Input: part model. Units: mm. Frame: model coordinates. A direction names the side the tool comes from. Round coordinates to 2 decimals unless told otherwise and drop trailing zeros. Loops run counter-clockwise (first coordinate to the right, second up) from the corner with the lowest first, then second, coordinate; pieces in that order, holes last. Notation, with made-up numbers: (0, 41) -> (34, 41) arc R7 cw to (34, 46) -> close; hole circle Ø1 at (36, 67.25). An arc over 180 degrees is marked (long way). Answer in a Markdown table with one row per item. Add a question column.
Q1. Ray query, L1, parallel to X at y = 61, z = 1; L2, parallel to Y at x = 25, z = 1.5; L3, parallel to Y at x = -42, z = 1.45. Return the intervals inside material, ascending. Write a range as from..to.
Q2. Section C-C, the plane y = 11.5. Output: boundary loops of the cut face in (x, z).
Q3. Section B-B, the plane y = 61.25. Output: boundary loops of the cut face in (x, z), and give its area (3 significant figures).
Q4. Mould query, pull axis Z, two halves, no side actions, for faces 1 (the face through (-11.15, -6.68, 25.87)), 2 (the face through (-30, 15, 25)), 3 (the face through (-26, 50, 5)). Classes: pulls with the +Z half, pulls with the -Z half, needs draft (parallel to the pull), parting line crosses it, or undercut.
Q5. Section D-D, the plane x = 15. Output: boundary loops of the cut face in (y, z).
Q6. Section A-A, the plane x = -10. Output: boundary loops of the cut face in (y, z).
Q7. Reachability of faces 4 (the face through (-67, 20, 2)), 5 (the face through (-17, 70, 7)), 6 (the face through (-75, 75, 2)) from +Z, -Z, +X, -X, +Y, -Y: full face, straight path, thin tool, end or side. Return the list, or none.
Q8. Pin query (flat end, axial travel): pin 1 (3.5 mm diameter, centred on y = 25, z = 9, fed in from -X); pin 2 (2 mm diameter, centred on x = -43, y = 17, fed in from +Z); pin 3 (2.5 mm diameter, centred on x = -28.5, y = 16.5, fed in from +Z). Return the tip coordinate at first contact, or that it passes through.
```python
from build123d import *

# Parameters (mm, degrees)
SKETCH_1_W               = 120
SKETCH_1_H               = 60
EXTRUDE_1_DEPTH          = 5
SKETCH_3_W               = 60
SKETCH_3_H               = 8
EXTRUDE_3_DEPTH          = 60
SKETCH_4_W               = 61.088110118
SKETCH_4_H               = 9
EXTRUDE_4_DEPTH          = 60
SKETCH_6_R               = 23.5
CUT_EXTRUDE_1_DEPTH      = 134.603892159
EXTRUDE_5_DEPTH          = 50
SKETCH_8_W               = 20.5
SKETCH_8_H               = 60.427303984
SKETCH_8_W_2             = 17.5
CUT_EXTRUDE_2_DEPTH      = 60
EXTRUDE_6_DEPTH          = 10
SKETCH_11_R              = 1.6
CUT_EXTRUDE_3_DEPTH      = 160.893337757
SKETCH_12_R              = 1.6
CUT_EXTRUDE_4_DEPTH      = 134.603892159
RIB_1_REACH              = 160.193
SKETCH_13_WALL_W         = 328.285335328
SKETCH_13_WALL_H         = 8
MIRROR_2_COPY_1_REACH    = 160.193
MIRROR_2_COPY_1_SKETCH_W = 328.285335328
MIRROR_2_COPY_1_SKETCH_H = 8
SKETCH_15_W              = 5
SKETCH_15_H              = 6.382962656
EXTRUDE_7_DEPTH          = 10
CHAMFER_2_SIZE           = 2
CHAMFER_3_SIZE           = 3
SKETCH_16_R              = 2.5
CUT_EXTRUDE_5_DEPTH      = 128.554500267
SKETCH_18_R              = 3.75
CUT_EXTRUDE_7_DEPTH      = 2


with BuildPart() as part:
    # 草图1 → 凸台-拉伸1 (new body)
    with BuildSketch(Plane.XY):
        with Locations((-25, 50)):
            Rectangle(SKETCH_1_W, SKETCH_1_H)
    extrude(amount=EXTRUDE_1_DEPTH)

    # 草图3 → 凸台-拉伸3 (add)
    with BuildSketch(Plane.XY.offset(5)):
        with Locations((5, 76)):
            Rectangle(SKETCH_3_W, SKETCH_3_H)
    extrude(amount=EXTRUDE_3_DEPTH)

    # 草图4 → 凸台-拉伸4 (add)
    with BuildSketch(Plane(origin=(35, 0, 0), x_dir=(0, 0, -1), z_dir=(1, 0, 0))):
        with Locations((-30.544055059, 18.117037344)):
            Rectangle(SKETCH_4_W, SKETCH_4_H)
    extrude(amount=-EXTRUDE_4_DEPTH)

    # 草图6 → 切除-拉伸1 (cut, through all)
    with BuildSketch(Plane(origin=(0, 0, 0), x_dir=(-1, 0, 0), z_dir=(0, 0, -1))):
        with Locations((-5, -9.213883343)):
            Circle(SKETCH_6_R)
    extrude(amount=-CUT_EXTRUDE_1_DEPTH, mode=Mode.SUBTRACT)

    # 草图7 → 凸台-拉伸5 (add)
    with BuildSketch(Plane(origin=(0, 0, 0), x_dir=(-1, 0, 0), z_dir=(0, 0, -1))):
        with BuildLine():
            Line((25, 13.617037344), (-35, 13.617037344))
            Line((-35, 13.617037344), (-35, -46.81026664))
            Line((-35, -46.81026664), (-28.815961295, -37.29636094))
            ThreePointArc((-28.815961295, -37.29636094), (-28.684669265, -37.061070002), (-28.586195427, -36.81026664))
            Line((-28.586195427, -36.81026664), (18.586195427, -36.81026664))
            ThreePointArc((18.586195427, -36.81026664), (18.684669265, -37.061070002), (18.815961295, -37.29636094))
            Line((18.815961295, -37.29636094), (25, -46.81026664))
            Line((25, -46.81026664), (25, 13.617037344))
        make_face()
    extrude(amount=-EXTRUDE_5_DEPTH)

    # 草图8 → 切除-拉伸2 (cut)
    with BuildSketch(Plane(origin=(35, 0, 0), x_dir=(0, 0, -1), z_dir=(1, 0, 0))):
        with Locations((-39.75, -16.596614648)):
            Rectangle(SKETCH_8_W, SKETCH_8_H)
        with Locations((-8.75, -16.596614648)):
            Rectangle(SKETCH_8_W_2, SKETCH_8_H)
    extrude(amount=-CUT_EXTRUDE_2_DEPTH, mode=Mode.SUBTRACT)

    # 草图9 → 凸台-拉伸6 (add)
    with BuildSketch(Plane.XZ.offset(-20)):
        with BuildLine():
            Line((-32.5, 0), (-41.5, 0))
            Line((-41.5, 0), (-44, 0))
            Line((-44, 0), (-44, 40))
            Line((-44, 40), (-41.5, 40))
            Line((-41.5, 40), (-41.5, 35.5))
            ThreePointArc((-41.5, 35.5), (-37, 31), (-32.5, 35.5))
            Line((-32.5, 35.5), (-32.5, 40))
            Line((-32.5, 40), (-30, 40))
            Line((-30, 40), (-30, 0))
            Line((-30, 0), (-32.5, 0))
        make_face()
    extrude(amount=EXTRUDE_6_DEPTH)

    # 草图11 → 切除-拉伸3 (cut, through all)
    with BuildSketch(Plane(origin=(0, 72, 0), x_dir=(-1, 0, 0), z_dir=(0, -1, 0))):
        with Locations(Location((-20, -52.088110118, 0), (0, 0, 90))):
            Circle(SKETCH_11_R)
        with Locations(Location((10, -28.088110118, 0), (0, 0, 90))):
            Circle(SKETCH_11_R)
        with Locations(Location((-20, -28.088110118, 0), (0, 0, 90))):
            Circle(SKETCH_11_R)
        with Locations(Location((10, -52.088110118, 0), (0, 0, 90))):
            Circle(SKETCH_11_R)
    extrude(amount=-CUT_EXTRUDE_3_DEPTH, mode=Mode.SUBTRACT)

    # 草图12 → 切除-拉伸4 (cut, through all)
    with BuildSketch(Plane(origin=(0, 0, 0), x_dir=(-1, 0, 0), z_dir=(0, 0, -1))):
        with Locations((42, 40.25)):
            Circle(SKETCH_12_R)
        with Locations((42, 61.25)):
            Circle(SKETCH_12_R)
        with Locations((72, 40.25)):
            Circle(SKETCH_12_R)
        with Locations((72, 61.25)):
            Circle(SKETCH_12_R)
    extrude(amount=-CUT_EXTRUDE_4_DEPTH, mode=Mode.SUBTRACT)

    # 草图13 wall → 筋1 (add, up to next)
    with BuildSketch(Plane(origin=(35, 68.5, 8.5), x_dir=(0, 0.707106781187, 0.707106781187), z_dir=(0, -0.707106781187, 0.707106781187)), mode=Mode.PRIVATE) as rib_1_sk1:
        with Locations((0, 4)):
            Rectangle(SKETCH_13_WALL_W, SKETCH_13_WALL_H)
    rib_1_tool1 = extrude(rib_1_sk1.sketch, amount=-RIB_1_REACH, mode=Mode.PRIVATE) - part.part
    rib_1 = rib_1_tool1.solids().sort_by_distance((35, 68.5, 8.5))[0]
    add(rib_1)

    # 镜向1: 筋1 across plane
    add(rib_1.mirror(Plane(origin=(5, 0, 0), x_dir=(0, 0, 1), z_dir=(1, 0, 0))))

    # 镜向2: 筋1 across plane
    add(rib_1.mirror(Plane(origin=(0, 47.308518672, 0), x_dir=(0, 0, 1), z_dir=(0, -1, 0))))

    # 镜向2 copy 1 sketch → 镜向2 copy 1 (add, up to next)
    with BuildSketch(Plane(origin=(-25, 26.117037344, 8.5), x_dir=(0, -0.7071067811870001, 0.7071067811869999), z_dir=(0, 0.7071067811869999, 0.7071067811870001)), mode=Mode.PRIVATE) as mirror_2_copy_1_sk1:
        with Locations((0, 4)):
            Rectangle(MIRROR_2_COPY_1_SKETCH_W, MIRROR_2_COPY_1_SKETCH_H)
    mirror_2_copy_1_tool1 = extrude(mirror_2_copy_1_sk1.sketch, amount=-MIRROR_2_COPY_1_REACH, mode=Mode.PRIVATE) - part.part
    add(mirror_2_copy_1_tool1.solids().sort_by_distance((-25, 26.117037344, 8.5))[0])

    # 草图15 → 凸台-拉伸7 (add)
    with BuildSketch(Plane(origin=(0, 0, 0), x_dir=(-1, 0, 0), z_dir=(0, 0, -1))):
        with Locations((27.5, 16.808518672)):
            Rectangle(SKETCH_15_W, SKETCH_15_H)
        with Locations((46.5, 16.808518672)):
            Rectangle(SKETCH_15_W, SKETCH_15_H)
    extrude(amount=-EXTRUDE_7_DEPTH)

    # 倒角2
    chamfer_2_edges = [part.edges().sort_by_distance(p)[0] for p in [
        (-49, 16.808518672, 10),
    ]]
    chamfer(chamfer_2_edges, length=CHAMFER_2_SIZE)

    # 倒角3
    chamfer_3_edges = [part.edges().sort_by_distance(p)[0] for p in [
        (-25, 76, 65),
        (35, 76, 65),
        (35, 18.117037344, 61.088110118),
        (-25, 18.117037344, 61.088110118),
    ]]
    chamfer(chamfer_3_edges, length=CHAMFER_3_SIZE)

    # 草图16 → 切除-拉伸5 (cut, through all)
    with BuildSketch(Plane(origin=(0, 22.617037344, 0), x_dir=(1, 0, 0), z_dir=(0, 1, 0))):
        with Locations(Location((20, -52.088110118, 0), (0, 0, 180))):
            Circle(SKETCH_16_R)
        with Locations(Location((-10, -52.088110118, 0), (0, 0, 180))):
            Circle(SKETCH_16_R)
        with Locations(Location((-10, -28.088110118, 0), (0, 0, 180))):
            Circle(SKETCH_16_R)
        with Locations(Location((20, -28.088110118, 0), (0, 0, 180))):
            Circle(SKETCH_16_R)
    extrude(amount=-CUT_EXTRUDE_5_DEPTH, mode=Mode.SUBTRACT)

    # 草图18 → 切除-拉伸7 (cut)
    with BuildSketch(Plane(origin=(0, 0, 0), x_dir=(-1, 0, 0), z_dir=(0, 0, -1))):
        with Locations((75, 75)):
            Circle(SKETCH_18_R)
        with Locations((25, 75)):
            Circle(SKETCH_18_R)
        with Locations((-25, 75)):
            Circle(SKETCH_18_R)
        with Locations((-25, 25)):
            Circle(SKETCH_18_R)
        with Locations((25, 25)):
            Circle(SKETCH_18_R)
        with Locations((75, 25)):
            Circle(SKETCH_18_R)
    extrude(amount=-CUT_EXTRUDE_7_DEPTH, mode=Mode.SUBTRACT)


solid = part.part
```
Answer block:
| question | item | result |
|---|---|---|
| 1 | L1 | -85..-73.58, -70.42..-43.58, -40.42..35 |
| 1 | L2 | 13.62..21.25, 28.75..71.25, 78.75..80 |
| 1 | L3 | 10..38.65, 41.85..59.65, 62.85..80 |
| 2 | outline | (-44, 0) -> (-30, 0) -> (-30, 40) -> (-32.5, 40) -> (-32.5, 35.5) arc R4.5 cw to (-41.5, 35.5) -> (-41.5, 40) -> (-44, 40) -> close; (-25, 17.5) -> (35, 17.5) -> (35, 29.5) -> (22.06, 29.5) arc R2.5 cw (long way) to (17.94, 29.5) -> (-7.94, 29.5) arc R2.5 cw (long way) to (-12.06, 29.5) -> (-25, 29.5) -> close |
| 3 | outline | (-85, 0) -> (-73.6, 0) -> (-73.6, 5) -> (-85, 5) -> close; (-70.4, 0) -> (-43.6, 0) -> (-43.6, 5) -> (-70.4, 5) -> close; (-40.4, 0) -> (35, 0) -> (35, 5) -> (-40.4, 5) -> close |
| 3 | area | 568 mm^2 |
| 4 | face 1 | undercut |
| 4 | face 2 | needs draft |
| 4 | face 3 | pulls with the +Z half |
| 5 | outline | (-36.81, 17.5) -> (13.62, 17.5) -> (13.62, 0) -> (80, 0) -> (80, 65) -> (72, 65) -> (72, 5) -> (22.62, 5) -> (22.62, 61.09) -> (13.62, 61.09) -> (13.62, 29.5) -> (-36.81, 29.5) -> close |
| 6 | outline | (-36.81, 17.5) -> (13.62, 17.5) -> (13.62, 0) -> (80, 0) -> (80, 26.49) -> (72, 26.49) -> (72, 5) -> (22.62, 5) -> (22.62, 25.59) -> (-36.81, 25.59) -> close; (13.62, 30.59) -> (22.62, 30.59) -> (22.62, 49.59) -> (13.62, 49.59) -> close; (13.62, 54.59) -> (22.62, 54.59) -> (22.62, 61.09) -> (13.62, 61.09) -> close; (72, 29.69) -> (80, 29.69) -> (80, 50.49) -> (72, 50.49) -> close; (72, 53.69) -> (80, 53.69) -> (80, 65) -> (72, 65) -> close |
| 7 | face 4 | +Z, -Z, -X, -Y |
| 7 | face 5 | +Z |
| 7 | face 6 | -Z |
| 8 | pin 1 | x = -25 |
| 8 | pin 2 | z = 40 |
| 8 | pin 3 | z = 10 |
